Could you check a few things on this model? Use its own coordinates, in mm. Face numbers are marked on the shaded views. A direction names the side the tool comes from. Give positions to 0.01 mm unless a question says otherwise; leave off trailing zeros. Loops run counter-clockwise (first coordinate to the right, second up) from the corner with the lowest first, then second, coordinate; pieces in that order, holes last.
1. For the marked faces 1 and 2, which set-ups out of +Z, -Z, +X, -X, +Y, -Y let a thin tool reach every point of the face, with its end or its side?
2. Imagine slicing it at A-A (z = 4). List the corners of the cut face in (x, y) for me, plus the area to 3 significant figures.
3. Imagine slicing it at B-B (y = 0). List the corners of the cut face in (x, z) for me, plus the area to 3 significant figures.
4. I need wall thicknesses on line 1 along X through (y, z) = (-7.5, 7); line 2 along X through (y, z) = (-10, 6); line 3 along Z through (x, y) = (-20, 19). Which ranges of each line are inside material? Lowest first, please.
5. For P1, Ø1.3, axis at x = 21, z = 8, coming from the -Y side; P2, Ø5, axis at x = 12.5, y = -28.5, coming from the +Z side; P3, Ø1.9, axis at y = -6, z = 8.5, coming from the +X side; P4, Ø2, axis at y = 25.5, z = 3.5, coming from the -X side, each with a flat end and sliding along its axis, tell me the tip position at first contact or that it passes through.
6. Imagine slicing it at D-D (x = -29.5). List the corners of the cut face in (y, z) for me, plus the area to 3 significant figures.
```python
from build123d import *

# Parameters (mm, degrees)
F0_R     = 38.1
F1_DEPTH = 1.27
F2_W     = 2.54
F2_H     = 2.54
F2_R     = 12.7
F3_DEPTH = 7.62


with BuildPart() as f1:
    # F0 (on Top) → F1 (new body)
    with BuildSketch(Plane.XY):
        Circle(F0_R)
    extrude(amount=F1_DEPTH)

    # F2 (on face) → F3 (join)
    with BuildSketch(Plane.XY.offset(1.27)):
        with Locations((21.616246, -6.438158)):
            Rectangle(F2_W, F2_H)
        Circle(F2_R)
    extrude(amount=F3_DEPTH)

    # F4 (on Front) → F5 (revolve)
    with BuildSketch(Plane.XZ):
        with BuildLine():
            Line((19.07809, 8.793222), (17.807475, 8.793222))
            ThreePointArc((17.807475, 8.793222), (21.616246, 5.08), (25.425016, 8.793222))
            Line((25.425016, 8.793222), (24.154401, 8.793222))
            ThreePointArc((24.154401, 8.793222), (21.616246, 6.35), (19.07809, 8.793222))
        make_face()
    revolve(axis=Axis((0, 0, 8.89), (0, 0, 1)))


solid = f1.part
```
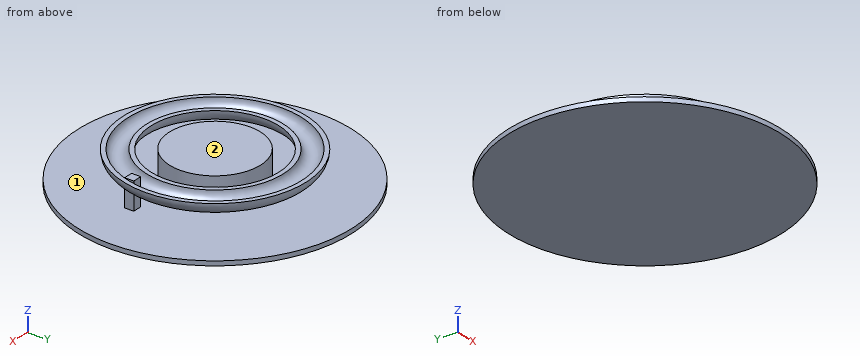
Derived:
1. face 1: none
1. face 2: +Z, +X, -X, +Y, -Y
2. outline: circle Ø25.4 at (0, 0); (20.35, -7.71) - (22.89, -7.71) - (22.89, -5.17) - (20.35, -5.17) - close
2. area: 513 mm2
3. outline: (-38.1, 0) - (38.1, 0) - (38.1, 1.27) - (12.7, 1.27) - (12.7, 8.89) - (-12.7, 8.89) - (-12.7, 1.27) - (-38.1, 1.27) - close; (-25.43, 8.79) arc R3.81 ccw to (-17.81, 8.79) - (-19.08, 8.79) arc R2.54 cw to (-24.15, 8.79) - close; (17.81, 8.79) arc R3.81 ccw to (25.43, 8.79) - (24.15, 8.79) arc R2.54 cw to (19.08, 8.79) - close
3. area: 315 mm2
4. line 1: x = -23.77 to -22.07, -18.45 to -16.7, -10.25 to 10.25, 16.7 to 18.45, 20.35 to 23.77
4. line 2: x = -21.93 to -16.31, -7.83 to 7.83, 16.31 to 21.93
4. line 3: z = 0 to 1.27
5. P1: stops at y = -15.1
5. P2: stops at z = 1.27
5. P3: stops at x = 24.91
5. P4: passes through
6. outline: (-24.11, 0) - (24.11, 0) - (24.11, 1.27) - (-24.11, 1.27) - close
6. area: 61.2 mm2
